Check sheet for the modelled part. Datum: model origin and axes. Units: mm. A direction names the side the tool comes from. Round coordinates to 2 decimals unless told otherwise and drop trailing zeros. Write each loop counter-clockwise with the first axis right and the second up, starting at its lowest first coordinate (ties: lowest second). Pieces come first, ordered by that corner, then holes. Notation, with made-up numbers: M 40,13 L 83,13 A25 cw 83,47 Z; hole C 63,20.5 d4. An arc over 180 degrees is marked long. One line per item, written item: value.
Autodesk Inventor part; units mm, degrees
ref_plane "YZ Plane" through (0, 0, 0) normal (1, 0, 0) x (0, 1, 0)
ref_plane "XZ Plane" through (0, 0, 0) normal (0, 1, 0) x (-1, 0, 0)
ref_plane "XY Plane" through (0, 0, 0) normal (0, 0, 1) x (1, 0, 0)
sketch "Sketch1" plane through (0, 0, 0) normal (0, 0, 1) x (1, 0, 0)
  line L0 (0, 6.16) -> (0, -6.16) construction
  line L1 (-6.16, 0) -> (6.16, 0) construction
  circle A0 centre (0, 0) radius 4.4
  circle A1 centre (0, 0) radius 2.5
  circle A2 centre (0, 3.5) radius 0.5
  line L2 (-2.25, -1.0897) -> (-2.25, -3.7812)
  line L3 (2.25, -1.0897) -> (2.25, -3.7812)
  point P0 (-2.25, -2.4355)
  dimension "d4" = 8.8
  dimension "d5" = 5
  dimension "d6" = 3.5
  dimension "d7" = 1
  dimension "d16" = 4.5
extrude "Extrusion3" add sketch "Sketch1" along normal blind 26 contours A0 L3 A1 L2 | A2 picked at (-2.534, -2.6638)
extrude "Extrusion4" add sketch "Sketch1" against normal blind 1.5 contours A2
chamfer "Chamfer1" distance 0.5 angle 45 4 edges at (0, 4.4, 0) (0, 2.5, 0) (0, 2.5, 26) (0, 4.4, 26)
chamfer "Chamfer2" distance 0.5 angle 45 2 edges at (2.25, -3.7812, 13) (-2.25, -3.7812, 13)
properties part number "Adjustment tool" material "ALMg4,5Mn-5083-(D54S)"
Q1. Access from +Z, -Z, +X, -X, +Y, -Y to the whole of each face (thin tool, end or side, straight path). Record for faces 1 (the cylindrical face through (0, 4, -1)), 2 (the flat face through (2.25, -2, 13)), 3 (the flat face through (0, 3.5, -1.5)).
Completed:
face 1: -Z
face 2: +Z, -Z, -Y
face 3: -Z, +X, -X, +Y, -Y
Q2. Draft check along Y on faces 4 (the cylindrical face through (-0.1, 2.5, 12.8)), 5 (the flat face through (-1, 3, 26)), 6 (the cylindrical face through (-0.153, 4.397, 12.825)). Enter one of: pulls with the +Y half, pulls with the -Y half, needs draft (parallel to the pull), parting line crosses it, or undercut.
Completed:
face 4: undercut
face 5: needs draft
face 6: parting line crosses it
Q3. Sectioned sample at A-A on y = 0. Enter the section's corners in (x, z).
Completed:
outline: M -4.4,0.5 L -3.9,0 L -3,0 L -2.5,0.5 L -2.5,25.5 L -3,26 L -3.9,26 L -4.4,25.5 Z; M 2.5,0.5 L 3,0 L 3.9,0 L 4.4,0.5 L 4.4,25.5 L 3.9,26 L 3,26 L 2.5,25.5 Z
Q4. Scan lines: line 1 (X direction, y = 0, z = 11.5); line 2 (Y direction, x = 0, z = 18.5); line 3 (X direction, y = 1.5, z = 0.75). Record each from-to range of solid material in increasing order. Write a range as [from, to].
Completed:
line 1: [-4.4, -2.5], [2.5, 4.4]
line 2: [2.5, 4.4]
line 3: [-4.14, -2], [2, 4.14]
Q5. Depth check by flat-ended pin: P1, Ø3, axis at x = -3, y = 1.5, coming from the -Z side; P2, Ø1.1, axis at y = -2.5, z = 8.5, coming from the -X side; P3, Ø0.7, axis at y = -2, z = 19, coming from the +X side. Enter the tip coordinate at first touch or a pass-through.
Completed:
P1: z = 0
P2: x = -3.94
P3: x = 4.08
